Part print with two shaded views. Sizes in mm from the minimum x, y, z corner. Round coordinates to 2 decimals unless told otherwise and drop trailing zeros. Loops run counter-clockwise (first coordinate to the right, second up) from the corner with the lowest first, then second, coordinate; pieces in that order, holes last. Notation, with made-up numbers: M 41,81.25 L 58,81.25 A17 ccw 58,96.25 Z; hole C 58,-10 d10. An arc over 180 degrees is marked long. Answer as CSV lines item,"result". Start each with the question number.
Item 1: Band-saw the part on A-A (y = 80). Give the cut face in (x, z).
Item 2: Band-saw the part on B-B (z = 0.8). Count the separate pieces of the cut face and the enclosed holes in it, and give its area (3 significant figures).
Item 3: Wall check: line 1 (X direction, y = 182, z = 2.4); line 2 (Y direction, x = 201, z = 2.5); line 3 (X direction, y = 132.5, z = 2.45). Give the ranges that are in metal, low to high.
Item 4: Band-saw the part on C-C (x = 149). Give the cut face in (y, z).
Item 5: Drop a flat-ended pin along its axis: pin 1 Ø4.5 at (x, y) = (9, 161.01) entering from -Z. Give the stop position or say it passes through.
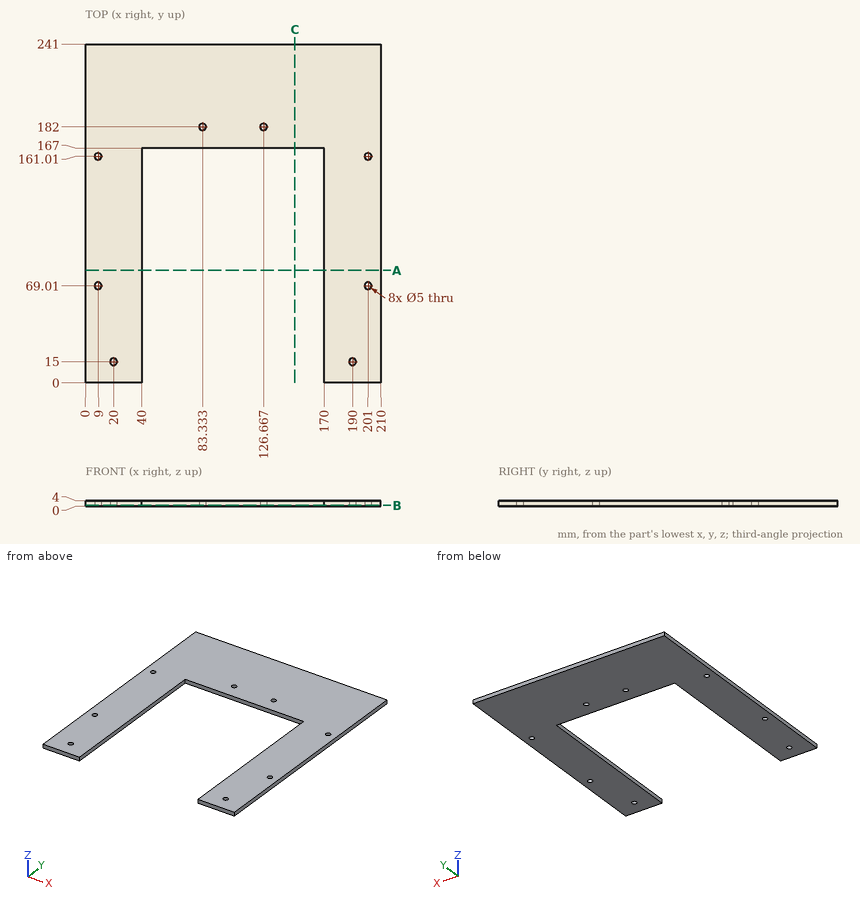
Answer block:
1,outline,"M 0,0 L 40,0 L 40,4 L 0,4 Z; M 170,0 L 210,0 L 210,4 L 170,4 Z"
2,separate pieces,"1"
2,enclosed holes,"8"
2,area,"28,700 mm^2"
3,line 1,"x = 0 to 80.83, 85.83 to 124.17, 129.17 to 210"
3,line 2,"y = 0 to 66.51, 71.51 to 158.51, 163.51 to 241"
3,line 3,"x = 0 to 40, 170 to 210"
4,outline,"M 167,0 L 241,0 L 241,4 L 167,4 Z"
5,pin 1,"passes through"
